Input: part model. Units: mm. Frame: model coordinates. Face numbers are marked on the shaded views. A direction names the side the tool comes from. Round coordinates to 2 decimals unless told otherwise and drop trailing zeros. Order: outer loops, then holes, each group sorted by start corner. A loop starts at its lowest first (then second) coordinate and runs counter-clockwise, first axis right, second up. Notation, with made-up numbers: (73, 51.25) -> (95, 51.25) arc R20 cw to (95, 72.25) -> close; hole circle Ø6 at (-15, 77). An arc over 180 degrees is marked (long way). Use a Markdown table: item, result.
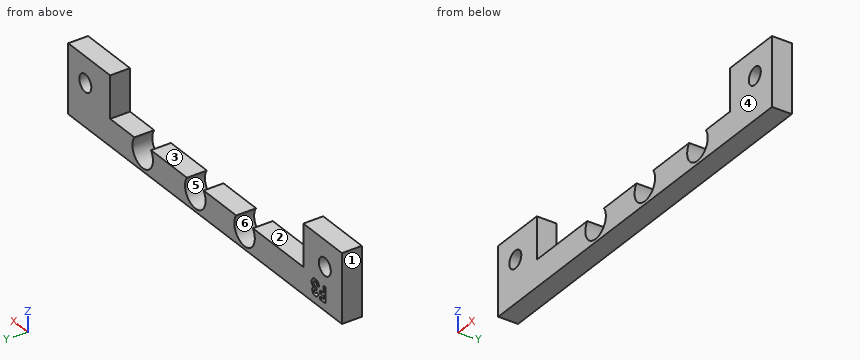
from build123d import *

# Parameters (mm, degrees)
BOSS_EXTRUDE1_OUTLINE_R = 1.75
BOSS_EXTRUDE1_DEPTH     = 4
CUT_EXTRUDE1_DEPTH      = 1


# Read off the part's stored shape, not the designer's step: Boss-Extrude1
with BuildPart() as part:
    # Boss-Extrude1 outline → Boss-Extrude1 (new body)
    with BuildSketch(Plane(origin=(0, 0, 0), x_dir=(1, 0, 0), z_dir=(0, 1, 0))):
        with BuildLine():
            Line((59.864776182, -18.81631321), (59.864776182, -4.977918302))
            Line((59.864776182, -4.977918302), (-20.135223818, -4.977918302))
            Line((-20.135223818, -4.977918302), (-20.135223818, -18.81631321))
            Line((-20.135223818, -18.81631321), (-8.860223818, -18.81631321))
            Line((-8.860223818, -18.81631321), (-8.860223818, -10.33743913))
            Line((-8.860223818, -10.33743913), (5.893075301, -10.33743913))
            ThreePointArc((5.893075301, -10.33743913), (8.329776182, -5.587442326), (10.766477064, -10.33743913))
            Line((10.766477064, -10.33743913), (20.283075301, -10.33743913))
            ThreePointArc((20.283075301, -10.33743913), (22.719776183, -5.587442326), (25.156477064, -10.33743913))
            Line((25.156477064, -10.33743913), (35.663075301, -10.33743913))
            ThreePointArc((35.663075301, -10.33743913), (38.099776182, -5.587442326), (40.536477064, -10.33743913))
            Line((40.536477064, -10.33743913), (47.599776182, -10.33743913))
            Line((47.599776182, -10.33743913), (47.599776182, -18.81631321))
            Line((47.599776182, -18.81631321), (59.864776182, -18.81631321))
        make_face()
        with Locations((-15.135223818, -13.587440845)):
            Circle(BOSS_EXTRUDE1_OUTLINE_R, mode=Mode.SUBTRACT)
        with Locations((54.864776182, -13.587440845)):
            Circle(BOSS_EXTRUDE1_OUTLINE_R, mode=Mode.SUBTRACT)
    extrude(amount=BOSS_EXTRUDE1_DEPTH)

    # Sketch2 → Cut-Extrude1 (cut)
    with BuildSketch(Plane(origin=(0, 4, 0), x_dir=(1, 0, 0), z_dir=(0, 1, 0))):
        Polygon((-15.320752279, -6.539659084), (-13.773957408, -6.539659084), (-13.773957408, -7.109530878), (-14.750880484, -7.109530878), (-14.750880484, -7.720107802), (-13.773957408, -7.720107802), (-13.773957408, -8.289979596), (-14.750880484, -8.289979596), (-14.750880484, -9.714659084), (-15.320752279, -9.714659084), align=None)
        with BuildLine():
            Line((-12.715624074, -7.31305652), (-13.285495869, -7.31305652))
            add(Edge.make_bspline(
                [(-13.285495869, -7.31305652), (-13.281472358, -7.284570661), (-13.27358453, -7.228726024), (-13.254710012, -7.1478769), (-13.232134053, -7.071185973), (-13.20394912, -6.998896107), (-13.17089278, -6.93087853), (-13.133301178, -6.86689984), (-13.090767935, -6.807234643), (-13.058165754, -6.771292092), (-13.041901118, -6.753361007)],
                knots=[0, 0, 0, 0, 1.111473889, 2.178970933, 3.205615836, 4.199322666, 5.174200091, 6.12565194, 7.064921805, 8, 8, 8, 8], degree=3))
            add(Edge.make_bspline(
                [(-13.041901118, -6.753361007), (-13.018441535, -6.729702238), (-12.972205164, -6.683073292), (-12.894938765, -6.623346763), (-12.813949309, -6.571657514), (-12.727612518, -6.530677903), (-12.637271857, -6.497509656), (-12.542208906, -6.475230469), (-12.442812126, -6.460448032), (-12.374986328, -6.458991911), (-12.340373674, -6.458248827)],
                knots=[0, 0, 0, 0, 1.01925491, 2.00884431, 2.983262333, 3.955970413, 4.92937149, 5.924503185, 6.940838805, 8, 8, 8, 8], degree=3))
            add(Edge.make_bspline(
                [(-12.340373674, -6.458248827), (-12.309601243, -6.458975304), (-12.249108846, -6.460403411), (-12.160200243, -6.471867479), (-12.07543333, -6.491974177), (-11.993912097, -6.518263234), (-11.916835455, -6.554033889), (-11.842502249, -6.595556006), (-11.772989349, -6.646484608), (-11.70813411, -6.704028804), (-11.648552204, -6.766268484), (-11.596954011, -6.832797584), (-11.55259412, -6.901838958), (-11.516047437, -6.973966208), (-11.487948004, -7.049301384), (-11.468446164, -7.127409284), (-11.455681736, -7.208117556), (-11.454410065, -7.262973882), (-11.4537651, -7.290795903)],
                knots=[0, 0, 0, 0, 1.091422571, 2.145516843, 3.172569842, 4.178562979, 5.178154469, 6.181868002, 7.194278174, 8.227918432, 9.254613415, 10.245994977, 11.209837596, 12.161663635, 13.10878368, 14.055455738, 15.013766427, 16, 16, 16, 16], degree=3))
            add(Edge.make_bspline(
                [(-11.4537651, -7.290795903), (-11.455088608, -7.325251158), (-11.457694188, -7.393082963), (-11.479074861, -7.492359849), (-11.512541427, -7.58728627), (-11.560887138, -7.67653406), (-11.62133159, -7.759860338), (-11.695494907, -7.834479257), (-11.781264727, -7.901560739), (-11.845653274, -7.937610336), (-11.878624876, -7.956070342)],
                knots=[0, 0, 0, 0, 0.992805628, 1.954529043, 2.915727527, 3.886831945, 4.871318353, 5.87440735, 6.911542536, 8, 8, 8, 8], degree=3))
            add(Edge.make_bspline(
                [(-11.878624876, -7.956070342), (-11.855993674, -7.963500642), (-11.811524378, -7.978100848), (-11.748316621, -8.006855789), (-11.688213266, -8.038280173), (-11.632249272, -8.074787023), (-11.57986801, -8.114900165), (-11.531388801, -8.1589625), (-11.486521994, -8.206877951), (-11.446000021, -8.258910035), (-11.410035187, -8.314226601), (-11.377765856, -8.371549868), (-11.351206398, -8.431749155), (-11.328707231, -8.494136944), (-11.311577646, -8.559273944), (-11.299516887, -8.626907755), (-11.292545473, -8.6968841), (-11.291482213, -8.744293031), (-11.290944587, -8.768264853)],
                knots=[0, 0, 0, 0, 1.059543567, 2.081955587, 3.086750234, 4.076226789, 5.052108497, 6.020845489, 6.989030705, 7.970690546, 8.952259656, 9.923888338, 10.895517021, 11.877585046, 12.873342345, 13.889638361, 14.932918083, 16, 16, 16, 16], degree=3))
            add(Edge.make_bspline(
                [(-11.290944587, -8.768264853), (-11.292034427, -8.803493698), (-11.294183369, -8.872957806), (-11.30784534, -8.975271328), (-11.333281467, -9.072818182), (-11.366744101, -9.16672079), (-11.411379623, -9.255766904), (-11.463908129, -9.342000012), (-11.528476217, -9.422429573), (-11.600232559, -9.499181935), (-11.679922161, -9.568961747), (-11.766318654, -9.629457703), (-11.857522252, -9.681373997), (-11.954109976, -9.723521124), (-12.056048269, -9.755979232), (-12.163109918, -9.779441448), (-12.275744768, -9.793796021), (-12.352626866, -9.795300826), (-12.391891101, -9.79606934)],
                knots=[0, 0, 0, 0, 1.005138573, 1.981928558, 2.936866704, 3.876260664, 4.820238198, 5.773547, 6.751179199, 7.756627054, 8.768222608, 9.766606018, 10.760583154, 11.757261445, 12.767156078, 13.807575856, 14.880313354, 16, 16, 16, 16], degree=3))
            add(Edge.make_bspline(
                [(-12.391891101, -9.79606934), (-12.429034435, -9.795259071), (-12.501663309, -9.793674698), (-12.607898237, -9.779961147), (-12.708864481, -9.757840075), (-12.804819707, -9.726658589), (-12.895392673, -9.686221532), (-12.98140473, -9.638070069), (-13.061139525, -9.579426938), (-13.135485462, -9.512939399), (-13.202793323, -9.438344155), (-13.2629507, -9.357369168), (-13.314631113, -9.269706524), (-13.358046503, -9.175730754), (-13.39285746, -9.075276996), (-13.420316241, -8.968549527), (-13.439496649, -8.855339836), (-13.445338083, -8.77744916), (-13.448316382, -8.737736007)],
                knots=[0, 0, 0, 0, 1.066544725, 2.085487077, 3.070979577, 4.031932826, 4.977951092, 5.916076795, 6.857635327, 7.814973522, 8.776389752, 9.738577119, 10.707772778, 11.69409279, 12.707140348, 13.757286496, 14.856535458, 16, 16, 16, 16], degree=3))
            Line((-13.448316382, -8.737736007), (-12.878444587, -8.737736007))
            add(Edge.make_bspline(
                [(-12.878444587, -8.737736007), (-12.874833369, -8.757704302), (-12.867799575, -8.796597793), (-12.85408059, -8.852906922), (-12.836202839, -8.904883726), (-12.815531711, -8.952990173), (-12.793203781, -8.997857884), (-12.766226302, -9.037829784), (-12.736576042, -9.073991275), (-12.693790501, -9.116980452), (-12.632625623, -9.161150038), (-12.550032773, -9.199535509), (-12.45815605, -9.222034111), (-12.393925058, -9.224778872), (-12.360726238, -9.226197545)],
                knots=[0, 0, 0, 0, 0.928156231, 1.807827665, 2.648129825, 3.438902246, 4.202261636, 4.936546065, 5.639352463, 6.338805438, 7.70633318, 9.064371875, 10.482673459, 12, 12, 12, 12], degree=3))
            add(Edge.make_bspline(
                [(-12.360726238, -9.226197545), (-12.34310977, -9.225895452), (-12.308603052, -9.225303719), (-12.257917821, -9.218745152), (-12.209633001, -9.207943188), (-12.163658661, -9.193263718), (-12.119702124, -9.174862085), (-12.078603224, -9.15113428), (-12.039524263, -9.12354732), (-12.002890065, -9.092532254), (-11.969039311, -9.058736934), (-11.940873493, -9.021314358), (-11.915131973, -8.983286333), (-11.896093359, -8.94216493), (-11.879411432, -8.900162922), (-11.869201241, -8.855755765), (-11.861491813, -8.809875003), (-11.861043772, -8.778476224), (-11.860816382, -8.762540694)],
                knots=[0, 0, 0, 0, 1.110435564, 2.175094844, 3.216326037, 4.226890168, 5.215276772, 6.21526065, 7.213097102, 8.228249917, 9.239874822, 10.221364777, 11.178138315, 12.128914389, 13.072518965, 14.022636769, 14.996447288, 16, 16, 16, 16], degree=3))
            add(Edge.make_bspline(
                [(-11.860816382, -8.762540694), (-11.86142006, -8.745112478), (-11.862621845, -8.710416892), (-11.872440552, -8.65978598), (-11.887946365, -8.611083124), (-11.909485835, -8.564524002), (-11.938249395, -8.520280222), (-11.972190076, -8.47746412), (-12.013981841, -8.438304198), (-12.059833004, -8.399595801), (-12.113002341, -8.365853754), (-12.170900429, -8.334714802), (-12.235048922, -8.30993781), (-12.303881896, -8.287807366), (-12.378701392, -8.271643634), (-12.459042809, -8.259907189), (-12.544776544, -8.251171225), (-12.603873921, -8.249917907), (-12.634213818, -8.249274468)],
                knots=[0, 0, 0, 0, 0.809814727, 1.612155564, 2.388397, 3.182215007, 3.988903953, 4.837162975, 5.715530372, 6.646997145, 7.623086902, 8.637258368, 9.698941581, 10.815059213, 11.996518529, 13.252603015, 14.589518788, 16, 16, 16, 16], degree=3))
            Line((-12.634213818, -8.249274468), (-12.634213818, -7.720107802))
            add(Edge.make_bspline(
                [(-12.634213818, -7.720107802), (-12.596438842, -7.716890764), (-12.525769343, -7.710872323), (-12.42767629, -7.69679799), (-12.345094583, -7.677985328), (-12.276039371, -7.655288868), (-12.218700348, -7.626140701), (-12.168609294, -7.593962412), (-12.125468509, -7.556592032), (-12.089008758, -7.51514394), (-12.059842092, -7.470632577), (-12.039199625, -7.423749779), (-12.025568418, -7.37594616), (-12.024276862, -7.343249925), (-12.023636895, -7.327048907)],
                knots=[0, 0, 0, 0, 1.70044513, 3.18119609, 4.440695891, 5.496282586, 6.431922213, 7.318171381, 8.16090191, 8.983045123, 9.787564368, 10.536848927, 11.275007137, 12, 12, 12, 12], degree=3))
            add(Edge.make_bspline(
                [(-12.023636895, -7.327048907), (-12.024741021, -7.306378167), (-12.026896043, -7.26603326), (-12.043633107, -7.208291197), (-12.072686755, -7.156818934), (-12.111642594, -7.111724783), (-12.159111639, -7.074058769), (-12.214753681, -7.046713885), (-12.277361285, -7.030647544), (-12.321409108, -7.028982006), (-12.344189779, -7.028120622)],
                knots=[0, 0, 0, 0, 1.009664648, 1.970651636, 2.907870547, 3.878035693, 4.867062054, 5.849714035, 6.887914197, 8, 8, 8, 8], degree=3))
            add(Edge.make_bspline(
                [(-12.344189779, -7.028120622), (-12.364837897, -7.029136964), (-12.405810086, -7.031153699), (-12.46572369, -7.046206069), (-12.522621653, -7.071544861), (-12.575325778, -7.106485562), (-12.623075271, -7.148447862), (-12.662263828, -7.198143497), (-12.694859012, -7.252595115), (-12.708675252, -7.29282371), (-12.715624074, -7.31305652)],
                knots=[0, 0, 0, 0, 0.98818071, 1.960853194, 2.938124878, 3.957524365, 4.978590984, 5.968022688, 6.978025184, 8, 8, 8, 8], degree=3))
        make_face()
    extrude(amount=-CUT_EXTRUDE1_DEPTH, mode=Mode.SUBTRACT)


solid = part.part
1) Line query: L1, parallel to X at y = 2, z = 13.5; L2, parallel to X at y = 3.75, z = 15.5; L3, parallel to X at y = 2.6, z = 6.75. Output: solid intervals per line, ascending. Write a range as [from, to].
Results found:
| item | result |
|---|---|
| L1 | x = [-20.14, -16.88], [-13.39, -8.86], [47.6, 53.12], [56.61, 59.86] |
| L2 | x = [-20.14, -8.86], [47.6, 59.86] |
| L3 | x = [-20.14, 5.96], [10.7, 20.35], [25.09, 35.73], [40.47, 59.86] |
2) Cut plane A-A on z = 16.75. Return loops of the section in (x, y).
Results found:
| item | result |
|---|---|
| outline | (-20.14, 0) -> (-8.86, 0) -> (-8.86, 4) -> (-20.14, 4) -> close; (47.6, 0) -> (59.86, 0) -> (59.86, 4) -> (47.6, 4) -> close |
3) Pin query (flat end, axial travel): pin 1 Ø5 at (x, z) = (8.33, 8.59) entering from -Y; pin 2 Ø2 at (x, y) = (16, 1.5) entering from +Z. Return the tip coordinate at first contact, or that it passes through.
Results found:
| item | result |
|---|---|
| pin 1 | passes through |
| pin 2 | stops at z = 10.34 |
4) Pull-direction query (Z, two-part tool) for the marked faces 3, 4, 5 and 6; classes: +Z half, -Z half, draft (parallel to the pull), parting line (faces both ways), or undercut.
Results found:
| item | result |
|---|---|
| face 3 | +Z half |
| face 4 | draft |
| face 5 | undercut |
| face 6 | undercut |
5) Cut plane C-C on z = 12.5. Return loops of the section in (x, y).
Results found:
| item | result |
|---|---|
| outline | (-20.14, 0) -> (-16.51, 0) -> (-16.51, 4) -> (-20.14, 4) -> close; (-13.76, 0) -> (-8.86, 0) -> (-8.86, 4) -> (-13.76, 4) -> close; (47.6, 0) -> (53.49, 0) -> (53.49, 4) -> (47.6, 4) -> close; (56.24, 0) -> (59.86, 0) -> (59.86, 4) -> (56.24, 4) -> close |
6) Cut plane D-D on x = 13.5. Return loops of the section in (y, z), and give its area (3 significant figures).
Results found:
| item | result |
|---|---|
| outline | (0, 4.98) -> (4, 4.98) -> (4, 10.34) -> (0, 10.34) -> close |
| area | 21.4 mm² |
7) Cut plane B-B on y = 1.2. Return loops of the section in (x, z), and give its area (3 significant figures).
Results found:
| item | result |
|---|---|
| outline | (-20.14, 4.98) -> (59.86, 4.98) -> (59.86, 18.82) -> (47.6, 18.82) -> (47.6, 10.34) -> (40.54, 10.34) arc R3 cw (long way) to (35.66, 10.34) -> (25.16, 10.34) arc R3 cw (long way) to (20.28, 10.34) -> (10.77, 10.34) arc R3 cw (long way) to (5.89, 10.34) -> (-8.86, 10.34) -> (-8.86, 18.82) -> (-20.14, 18.82) -> close; hole circle Ø3.5 at (-15.14, 13.59); hole circle Ø3.5 at (54.86, 13.59) |
| area | 537 mm² |
8) Set-up query: the marked faces 1 and 2. Return all of +Z, -Z, +X, -X, +Y, -Y with unobstructed straight access to the full face (end or side cutting, diameter ignored); none if empty.
Results found:
| item | result |
|---|---|
| face 1 | +Z, -Z, -X, +Y, -Y |
| face 2 | +Z, +Y, -Y |
